The model under review builds one solid part; all positions refer to its coordinate system, in mm. Face numbers are marked on the shaded views. Round coordinates to 2 decimals unless told otherwise and drop trailing zeros. Order: outer loops, then holes, each group sorted by start corner. A loop starts at its lowest first (then second) coordinate and runs counter-clockwise, first axis right, second up.
1) Clearance check with flat-ended pins moving along their axes: P1, Ø1.5, axis at y = -10, z = -18.5, coming from the -X side; P2, Ø3, axis at y = -9.5, z = -24, coming from the +X side; P3, Ø5, axis at x = 3.5, y = -10, coming from the -Z side. State where each tip first meets the part, or that it passes through.
2) Consider section C-C (y = -1.75). Give the number of separate pieces and of enclosed holes in the cut face, then the cut area to 3 significant figures.
3) To check wall thickness, follow L1, parallel to Z at x = 14.5, y = -11.75; L2, parallel to Z at x = -2.5, y = -10.5; L3, parallel to X at y = -11.75, z = -22. State the ranges of each line that lie inside material, in increasing order.
4) Mouldability with a two-part tool opening along Z and no side actions: class the marked faces 1, 2 and 3 as pulls with the +Z half, pulls with the -Z half, needs draft (parallel to the pull), parting line crosses it, or undercut.
5) Consider section A-A (z = -25). Give the boundary of the cut face in (x, y), then the cut area to 3 significant figures.
6) Consider section B-B (x = 13). Give the boundary of the cut face in (y, z), then the cut area to 3 significant figures.
7) Consider section D-D (z = 25.5). Give the boundary of the cut face in (x, y).
from build123d import *

# Parameters (mm, degrees)
F0_R     = 34.925
F0_R_2   = 3.175
F1_DEPTH = 12.7


with BuildPart() as f1:
    # F0 (on Front) → F1 (new body)
    with BuildSketch(Plane.XZ):
        Circle(F0_R)
        with Locations((-0.247554, -27.350496)):
            Circle(F0_R_2, mode=Mode.SUBTRACT)
        with Locations((-13.889636, -23.562447)):
            Circle(F0_R_2, mode=Mode.SUBTRACT)
        with Locations((-23.810001, -13.46086)):
            Circle(F0_R_2, mode=Mode.SUBTRACT)
        with Locations((13.46086, -23.810001)):
            Circle(F0_R_2, mode=Mode.SUBTRACT)
        with Locations((23.562447, -13.889636)):
            Circle(F0_R_2, mode=Mode.SUBTRACT)
        with Locations((27.350496, -0.247554)):
            Circle(F0_R_2, mode=Mode.SUBTRACT)
        with Locations((-27.350496, 0.247554)):
            Circle(F0_R_2, mode=Mode.SUBTRACT)
        with Locations((-23.562447, 13.889636)):
            Circle(F0_R_2, mode=Mode.SUBTRACT)
        with Locations((-13.46086, 23.810001)):
            Circle(F0_R_2, mode=Mode.SUBTRACT)
        with Locations((23.810001, 13.46086)):
            Circle(F0_R_2, mode=Mode.SUBTRACT)
        with Locations((13.889636, 23.562447)):
            Circle(F0_R_2, mode=Mode.SUBTRACT)
        with Locations((0.247554, 27.350496)):
            Circle(F0_R_2, mode=Mode.SUBTRACT)
    extrude(amount=F1_DEPTH)


solid = f1.part
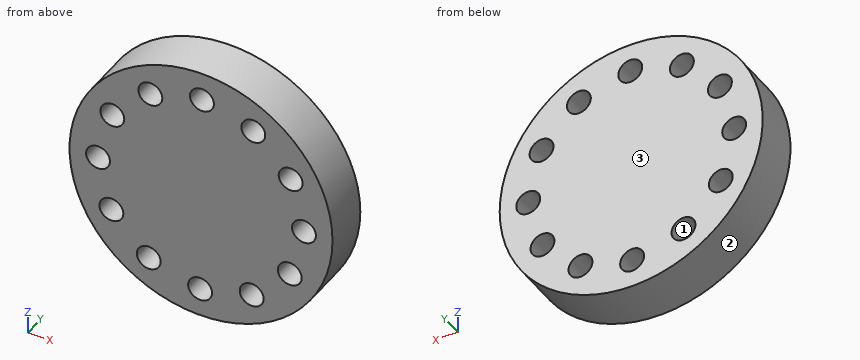
Answer below:
1. P1: stops at x = -30.08
1. P2: stops at x = 26.71
1. P3: stops at z = -34.91
2. separate pieces: 1
2. enclosed holes: 12
2. area: 3,450 mm2
3. L1: z = -31.77 to -26.81, -20.81 to 20.45, 26.68 to 31.77
3. L2: z = -34.84 to -29.59, -25.11 to 25.76, 28.94 to 34.84
3. L3: x = -27.12 to -16.65, -11.13 to 10.85, 16.07 to 27.12
4. face 1: undercut
4. face 2: parting line crosses it
4. face 3: needs draft
5. outline: (-24.39, -12.7) - (-16.72, -12.7) - (-16.72, 0) - (-24.39, 0) - close; (-11.06, -12.7) - (-2.38, -12.7) - (-2.38, 0) - (-11.06, 0) - close; (1.89, -12.7) - (10.52, -12.7) - (10.52, 0) - (1.89, 0) - close; (16.4, -12.7) - (24.39, -12.7) - (24.39, 0) - (16.4, 0) - close
5. area: 419 mm2
6. outline: (-12.7, -32.42) - (0, -32.42) - (0, -26.95) - (-12.7, -26.95) - close; (-12.7, -20.67) - (0, -20.67) - (0, 20.51) - (-12.7, 20.51) - close; (-12.7, 26.61) - (0, 26.61) - (0, 32.42) - (-12.7, 32.42) - close
6. area: 666 mm2
7. outline: (-23.86, -12.7) - (-16.15, -12.7) - (-16.15, 0) - (-23.86, 0) - close; (-10.77, -12.7) - (-2.33, -12.7) - (-2.33, 0) - (-10.77, 0) - close; (2.83, -12.7) - (11.37, -12.7) - (11.37, 0) - (2.83, 0) - close; (16.4, -12.7) - (23.86, -12.7) - (23.86, 0) - (16.4, 0) - close
